The model under review builds one solid part; all positions refer to its coordinate system, in mm. Face numbers are marked on the shaded views. A direction names the side the tool comes from. Coordinates: 2 decimals unless noted, no trailing zeros. Order: outer loops, then holes, each group sorted by start corner. A loop starts at its lowest first (then second) coordinate and runs counter-clockwise, first axis right, second up.
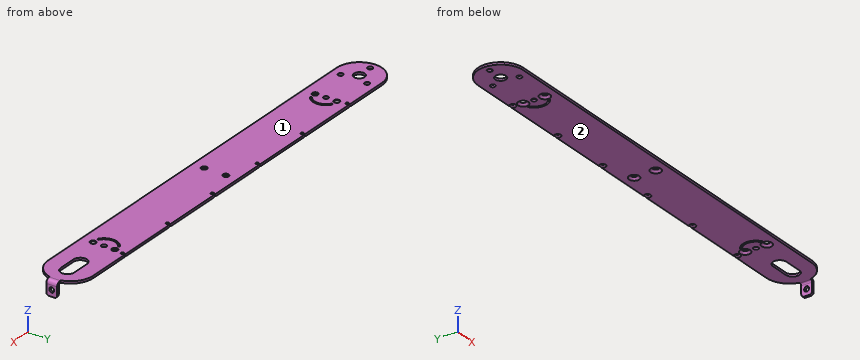
```python
from build123d import *

# Parameters (mm, degrees)
AUFSATZ_LINEAR_START                        = -96.5
AUFSATZ_LINEAR_AUSTRAGEN1_DEPTH             = 2.5
SKIZZE3_W                                   = 2.5
SKIZZE3_H                                   = 6
AUFSATZ_LINEAR_AUSTRAGEN2_DEPTH             = 14
VERRUNDUNG1_R                               = 3
DURCHGANGSLOCH_F_R_M51_D                    = 5.5
KREISMUSTER1_COUNT                          = 3
DURCHGANGSLOCH_F_R_M5_EINSTELLSCHRAUBE_D    = 5.5
VOLUMENK_RPER_START                         = -6
VOLUMENK_RPER_UMWANDELN2_DEPTH              = 12
VOLUMENK_RPER_UMWANDELN2_2_DEPTH            = 12
FORMSENKUNG_F_R_M3_SENKSCHRAUBE_MIT_2_COUNT = 2
FORMSENKUNG_F_R_M3_SENKSCHRAUBE_MIT_2_PITCH = 70
FORMSENKUNG_F_R_M3_SENKSCHRAUBE_MIT_3_COUNT = 2
FORMSENKUNG_F_R_M3_SENKSCHRAUBE_MIT_3_PITCH = 140
FORMSENKUNG_F_R_M3_SENKSCHRAUBE_MIT_4_COUNT = 2
FORMSENKUNG_F_R_M3_SENKSCHRAUBE_MIT_4_PITCH = 210
FORMSENKUNG_F_R_M3_SENKSCHRAUBE_MIT_5_COUNT = 2
FORMSENKUNG_F_R_M3_SENKSCHRAUBE_MIT_5_PITCH = 280
FORMSENKUNG_F_R_M3_SENKSCHRAUBE_MIT_6_COUNT = 2
FORMSENKUNG_F_R_M3_SENKSCHRAUBE_MIT_6_PITCH = 350
FORMSENKUNG_F_R_M5_SENKSCHRAUBE_MIT_2_COUNT = 2
FORMSENKUNG_F_R_M5_SENKSCHRAUBE_MIT_2_PITCH = 173
DURCHGANGSLOCH_F_R_M52_D                    = 5.5
SCHNITT_LINEAR_AUSTRAGEN1_REACH             = 482.355


# Read off the part's stored shape, not the designer's step: Volumenkörper umwandeln2
with BuildPart() as part:
    # Skizze1 → Aufsatz-Linear austragen1 (new body)
    with BuildSketch(Plane.XY.offset(AUFSATZ_LINEAR_START)):
        with BuildLine():
            Line((462.5, 0), (475, 0))
            Line((475, 0), (477, 0))
            Line((477, 0), (479.5, 0))
            Line((479.5, 0), (479.5, 6))
            Line((479.5, 6), (474.269322199, 6))
            ThreePointArc((474.269322199, 6), (465.411035007, 19.685019685), (450, 25))
            Line((450, 25), (0, 25))
            ThreePointArc((0, 25), (-17.67766953, 17.67766953), (-25, 0))
            Line((-25, 0), (-6, 0))
            ThreePointArc((-6, 0), (0, 6), (6, 0))
            Line((6, 0), (427.5, 0))
            ThreePointArc((427.5, 0), (429.696699141, 5.303300859), (435, 7.5))
            Line((435, 7.5), (450, 7.5))
            Line((450, 7.5), (455, 7.5))
            ThreePointArc((455, 7.5), (460.303300859, 5.303300859), (462.5, 0))
        make_face()
    extrude(amount=-AUFSATZ_LINEAR_AUSTRAGEN1_DEPTH)

    # Skizze3 → Aufsatz-Linear austragen2 (add)
    with BuildSketch(Plane(origin=(0, 0, -99), x_dir=(-1, 0, 0), z_dir=(0, 0, -1))):
        with Locations((-478.25, 3)):
            Rectangle(SKIZZE3_W, SKIZZE3_H)
    extrude(amount=AUFSATZ_LINEAR_AUSTRAGEN2_DEPTH)

    # Verrundung1
    verrundung1_edges = [part.edges().sort_by_distance(p)[0] for p in [
        (478.25, 6, -113),
    ]]
    fillet(verrundung1_edges, radius=VERRUNDUNG1_R)

    # Spiegeln1: part across plane


with BuildPart() as part_1:
    add(part.part)
    add(part.part.mirror(Plane(origin=(6, 0, -99), x_dir=(0, 0, 1), z_dir=(0, -1, 0))))

    # Durchgangsloch für M51 (through all)
    with Locations(Plane(origin=(0, 0, -99), x_dir=(-1, 0, 0), z_dir=(0, 0, -1))):
        with Locations((17, 0)):
            durchgangsloch_f_r_m51 = Hole(DURCHGANGSLOCH_F_R_M51_D / 2)

    # Kreismuster1: Durchgangsloch für M51 ×3 about axis
    kreismuster1_axis = Axis((0, 0, 0), (0, 0, 1))
    for i in range(1, KREISMUSTER1_COUNT):
        add(durchgangsloch_f_r_m51.rotate(kreismuster1_axis, i * 360 / KREISMUSTER1_COUNT), mode=Mode.SUBTRACT)

    # Durchgangsloch für M5 Einstellschraube (through all)
    with Locations(Plane(origin=(479.5, 0, 0), x_dir=(0, 0, -1), z_dir=(1, 0, 0))):
        with Locations((106, 0)):
            Hole(DURCHGANGSLOCH_F_R_M5_EINSTELLSCHRAUBE_D / 2)

    # Volumenkörper umwandeln2 outline → Volumenkörper umwandeln2 (cut)
    with BuildSketch(Plane(origin=(0, 0, 0), x_dir=(1, 0, 0), z_dir=(0, 1, 0)).offset(VOLUMENK_RPER_START)):
        with BuildLine():
            Line((479.5, 96.5), (479.5, 101))
            ThreePointArc((479.5, 101), (478.181980515, 97.818019485), (475, 96.5))
            Line((475, 96.5), (479.5, 96.5))
        make_face()
    extrude(amount=VOLUMENK_RPER_UMWANDELN2_DEPTH, mode=Mode.SUBTRACT)

    # Volumenk_rper umwandeln2 2 outline → Volumenk_rper umwandeln2 2 (add)
    with BuildSketch(Plane(origin=(0, 0, 0), x_dir=(1, 0, 0), z_dir=(0, 1, 0)).offset(VOLUMENK_RPER_START)):
        with BuildLine():
            Line((477, 99), (477, 101))
            ThreePointArc((477, 101), (476.414213562, 99.585786438), (475, 99))
            Line((475, 99), (477, 99))
        make_face()
    extrude(amount=VOLUMENK_RPER_UMWANDELN2_2_DEPTH)

    # Skizze13 → Formsenkung für M3 Senkschraube mit Innensechskant1 (revolve, cut)
    with BuildSketch(Plane(origin=(400, 22, -99), x_dir=(0, 1, 0), z_dir=(1, 0, 0))):
        Polygon((0, 0), (0, 2.5), (1.7, 2.5), (1.7, 1.77), (3.47, 0), align=None)
    formsenkung_f_r_m3_senkschraube_mit_inne = revolve(axis=Axis((400, 22, -105.35), (0, 0, 1)), mode=Mode.SUBTRACT)

    # Formsenkung f_r M3 Senkschraube mit  2: Formsenkung für M3 Senkschraube mit Innensechskant1 ×2
    with Locations(*[(-i * FORMSENKUNG_F_R_M3_SENKSCHRAUBE_MIT_2_PITCH, 0, 0) for i in range(1, FORMSENKUNG_F_R_M3_SENKSCHRAUBE_MIT_2_COUNT)]):
        add(formsenkung_f_r_m3_senkschraube_mit_inne, mode=Mode.SUBTRACT)

    # Formsenkung f_r M3 Senkschraube mit  3: Formsenkung für M3 Senkschraube mit Innensechskant1 ×2
    with Locations(*[(-i * FORMSENKUNG_F_R_M3_SENKSCHRAUBE_MIT_3_PITCH, 0, 0) for i in range(1, FORMSENKUNG_F_R_M3_SENKSCHRAUBE_MIT_3_COUNT)]):
        add(formsenkung_f_r_m3_senkschraube_mit_inne, mode=Mode.SUBTRACT)

    # Formsenkung f_r M3 Senkschraube mit  4: Formsenkung für M3 Senkschraube mit Innensechskant1 ×2
    with Locations(*[(-i * FORMSENKUNG_F_R_M3_SENKSCHRAUBE_MIT_4_PITCH, 0, 0) for i in range(1, FORMSENKUNG_F_R_M3_SENKSCHRAUBE_MIT_4_COUNT)]):
        add(formsenkung_f_r_m3_senkschraube_mit_inne, mode=Mode.SUBTRACT)

    # Formsenkung f_r M3 Senkschraube mit  5: Formsenkung für M3 Senkschraube mit Innensechskant1 ×2
    with Locations(*[(-i * FORMSENKUNG_F_R_M3_SENKSCHRAUBE_MIT_5_PITCH, 0, 0) for i in range(1, FORMSENKUNG_F_R_M3_SENKSCHRAUBE_MIT_5_COUNT)]):
        add(formsenkung_f_r_m3_senkschraube_mit_inne, mode=Mode.SUBTRACT)

    # Formsenkung f_r M3 Senkschraube mit  6: Formsenkung für M3 Senkschraube mit Innensechskant1 ×2
    with Locations(*[(-i * FORMSENKUNG_F_R_M3_SENKSCHRAUBE_MIT_6_PITCH, 0, 0) for i in range(1, FORMSENKUNG_F_R_M3_SENKSCHRAUBE_MIT_6_COUNT)]):
        add(formsenkung_f_r_m3_senkschraube_mit_inne, mode=Mode.SUBTRACT)

    # Skizze15 → Formsenkung für M5 Senkschraube mit Innensechskant1 (revolve, cut)
    with BuildSketch(Plane(origin=(52, 12, -99), x_dir=(0, 1, 0), z_dir=(1, 0, 0))):
        Polygon((0, 0), (0, 2.5), (2.75, 2.5), (2.75, 2.985), (5.735, 0), align=None)
    formsenkung_f_r_m5_senkschraube_mit_inne = revolve(axis=Axis((52, 12, -105.35), (0, 0, 1)), mode=Mode.SUBTRACT)

    # Formsenkung f_r M5 Senkschraube mit  2: Formsenkung für M5 Senkschraube mit Innensechskant1 ×2
    with Locations(*[(i * FORMSENKUNG_F_R_M5_SENKSCHRAUBE_MIT_2_PITCH, 0, 0) for i in range(1, FORMSENKUNG_F_R_M5_SENKSCHRAUBE_MIT_2_COUNT)]):
        add(formsenkung_f_r_m5_senkschraube_mit_inne, mode=Mode.SUBTRACT)

    # Spiegeln2: Formsenkung für M5 Senkschraube mit Innensechskant1 across plane
    add(formsenkung_f_r_m5_senkschraube_mit_inne.mirror(Plane(origin=(225, 0, 0), x_dir=(0, 0, 1), z_dir=(1, 0, 0))), mode=Mode.SUBTRACT)

    # Spiegeln2 copy 1 sketch → Spiegeln2 copy 1 (revolve, cut)
    with BuildSketch(Plane(origin=(225, 12, -99), x_dir=(0, 1, 0), z_dir=(-1, 0, 0))):
        Polygon((0, 0), (0, -2.5), (2.75, -2.5), (2.75, -2.985), (5.735, 0), align=None)
    revolve(axis=Axis((225, 12, -105.35), (0, 0, -1)), mode=Mode.SUBTRACT)

    # Spiegeln2 at the second plane: Formsenkung für M5 Senkschraube mit Innensechskant1 across plane
    add(formsenkung_f_r_m5_senkschraube_mit_inne.mirror(Plane.ZX), mode=Mode.SUBTRACT)

    # Spiegeln2 at the second plane copy 1 ske → Spiegeln2 at the second plane copy 1 (revolve, cut)
    with BuildSketch(Plane(origin=(225, -12, -99), x_dir=(0, -1, 0), z_dir=(1, 0, 0))):
        Polygon((0, 0), (0, -2.5), (2.75, -2.5), (2.75, -2.985), (5.735, 0), align=None)
    revolve(axis=Axis((225, -12, -105.35), (0, 0, -1)), mode=Mode.SUBTRACT)

    # Spiegeln2 at the second plane copy 2 ske → Spiegeln2 at the second plane copy 2 (revolve, cut)
    with BuildSketch(Plane(origin=(398, -12, -99), x_dir=(0, -1, 0), z_dir=(-1, 0, 0))):
        Polygon((0, 0), (0, 2.5), (2.75, 2.5), (2.75, 2.985), (5.735, 0), align=None)
    revolve(axis=Axis((398, -12, -105.35), (0, 0, 1)), mode=Mode.SUBTRACT)

    # Spiegeln2 at the second plane copy 3 ske → Spiegeln2 at the second plane copy 3 (revolve, cut)
    with BuildSketch(Plane(origin=(225, -12, -99), x_dir=(0, -1, 0), z_dir=(-1, 0, 0))):
        Polygon((0, 0), (0, 2.5), (2.75, 2.5), (2.75, 2.985), (5.735, 0), align=None)
    revolve(axis=Axis((225, -12, -105.35), (0, 0, 1)), mode=Mode.SUBTRACT)

    # Durchgangsloch für M52 (through all)
    with Locations(Plane(origin=(0, 0, -99), x_dir=(-1, 0, 0), z_dir=(0, 0, -1))):
        with Locations((-52, 0)):
            durchgangsloch_f_r_m52 = Hole(DURCHGANGSLOCH_F_R_M52_D / 2)

    # Skizze19 → Schnitt-Linear austragen1 (cut, up to next)
    with BuildSketch(Plane(origin=(0, 0, -99), x_dir=(-1, 0, 0), z_dir=(0, 0, -1)), mode=Mode.PRIVATE) as schnitt_linear_austragen1_sk1:
        with BuildLine():
            Line((-59.155963734, -12.611192768), (-57.924777873, -11.006680115))
            ThreePointArc((-57.924777873, -11.006680115), (-64.5, 0), (-57.924777873, 11.006680115))
            Line((-57.924777873, 11.006680115), (-59.155963734, 12.611192768))
            ThreePointArc((-59.155963734, 12.611192768), (-60.01066697, 12.086323457), (-60.827040721, 11.503623434))
            ThreePointArc((-60.827040721, 11.503623434), (-66.5, 0), (-60.827040721, -11.503623434))
            ThreePointArc((-60.827040721, -11.503623434), (-60.01066697, -12.086323457), (-59.155963734, -12.611192768))
        make_face()
    schnitt_linear_austragen1_tool1 = extrude(schnitt_linear_austragen1_sk1.sketch, amount=-SCHNITT_LINEAR_AUSTRAGEN1_REACH, mode=Mode.PRIVATE) & part_1.part
    schnitt_linear_austragen1 = schnitt_linear_austragen1_tool1.solids().sort_by_distance((59.86349, -11.864266, -99))[0]
    add(schnitt_linear_austragen1, mode=Mode.SUBTRACT)

    # Spiegeln3: Durchgangsloch für M52, Schnitt-Linear austragen1 across plane
    add(durchgangsloch_f_r_m52.mirror(Plane(origin=(225, 0, 0), x_dir=(0, 0, 1), z_dir=(1, 0, 0))), mode=Mode.SUBTRACT)
    add(schnitt_linear_austragen1.mirror(Plane(origin=(225, 0, 0), x_dir=(0, 0, 1), z_dir=(1, 0, 0))), mode=Mode.SUBTRACT)


solid = part_1.part
```
(1) Machinability: for the marked faces 1 and 2, which of the approach directions +Z, -Z, +X, -X, +Y, -Y give a long, thin tool a straight path to every point of the face, cutting with its end or side? Answer none if there is none.
A:
face 1: +Z, +X, -X, +Y, -Y
face 2: -Z, -X, +Y, -Y
(2) We need section B-B, the plane x = 182. Write out the cut boundary in (y, z).
A:
outline: (-25, -99) - (25, -99) - (25, -96.5) - (-25, -96.5) - close
(3) We need section A-A, the plane x = 442. Write out the cut boundary in (y, z), and give its area (3 significant figures).
A:
outline: (-25, -99) - (-7.5, -99) - (-7.5, -96.5) - (-25, -96.5) - close; (7.5, -99) - (25, -99) - (25, -96.5) - (7.5, -96.5) - close
area: 87.5 mm2
(4) Wall thickness on probe 1 along Y at (x, z) = (260, -97); probe 2 along Z at (x, y) = (419, -6); probe 3 along X at (y, z) = (5, -109.5): over which ranges is each line inside the solid? List them lowest first.
A:
probe 1: y = -25 to 20.3, 23.7 to 25
probe 2: z = -99 to -96.5
probe 3: x = 477 to 479.5
(5) For pin 1 Ø6 at (y, z) = (-1.5, -107) entering from -X; pin 2 Ø4 at (x, z) = (476, -103.5) entering from -Y; pin 3 Ø4.5 at (x, y) = (52, 0) entering from -Z; pin 4 Ø9 at (x, y) = (8.5, -14.72) entering from -Z, all flat-tipped, find the tip position at first contact; note any pin that passes through.
A:
pin 1: stops at x = 477
pin 2: stops at y = -6
pin 3: passes through
pin 4: stops at z = -99
